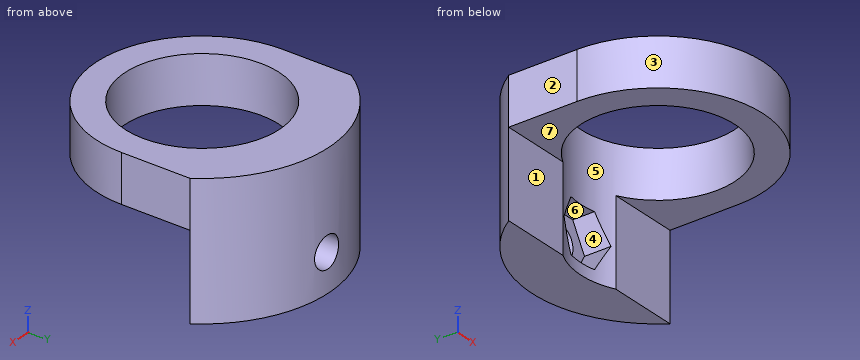
```python
from build123d import *

# Parameters (mm, degrees)
SKETCH1_R               = 8.1
BOSS_EXTRUDE1_DEPTH     = 14
CUT_EXTRUDE1_REACH      = 31.401
SKETCH2_W               = 9
SKETCH2_H               = 18.335502747
CUT_EXTRUDE2_REACH      = 27.601
CUT_EXTRUDE2_END_RADIUS = 13.25
SKETCH3_R               = 1.65
CUT_EXTRUDE3_DEPTH      = 3


with BuildPart() as part:
    # Sketch1 → Boss-Extrude1 (new body)
    with BuildSketch(Plane.XY):
        with BuildLine():
            ThreePointArc((-11.1, 0), (0, -11.1), (11.1, 0))
            Line((11.1, 0), (11.1, 7.235502747))
            ThreePointArc((11.1, 7.235502747), (0, 13.25), (-11.1, 7.235502747))
            Line((-11.1, 7.235502747), (-11.1, 0))
        make_face()
        Circle(SKETCH1_R, mode=Mode.SUBTRACT)
    extrude(amount=BOSS_EXTRUDE1_DEPTH)

    # Cut-Extrude1: up to this face of the body (flat: up to its plane)
    cut_extrude1_end = Plane(part.part.faces().sort_by_distance((11.1, 3.617751373, 7))[0])
    # Sketch2 → Cut-Extrude1 (cut, up to the picked face)
    with BuildSketch(Plane.ZY.offset(11.1), mode=Mode.PRIVATE) as cut_extrude1_sk1:
        with Locations((4.5, -1.932248627)):
            Rectangle(SKETCH2_W, SKETCH2_H)
    cut_extrude1_tool1 = split(extrude(cut_extrude1_sk1.sketch, amount=-CUT_EXTRUDE1_REACH, mode=Mode.PRIVATE), bisect_by=cut_extrude1_end, keep=Keep.BOTH, mode=Mode.PRIVATE)
    add(cut_extrude1_tool1.solids().sort_by(Axis((-11.1, -1.932249, 4.5), (1, 0, 0)))[0], mode=Mode.SUBTRACT)

    # Cut-Extrude2: up to this cylinder (the profile starts inside it)
    cut_extrude2_end = Plane(origin=(0, 0, 4), z_dir=(0, 0, -1)) * Cylinder(CUT_EXTRUDE2_END_RADIUS, 82.702, mode=Mode.PRIVATE)
    # Sketch3 → Cut-Extrude2 (cut, up to the surface)
    with BuildSketch(Plane.XZ.offset(-7.235502747), mode=Mode.PRIVATE) as cut_extrude2_sk1:
        with Locations((0, 4)):
            Circle(SKETCH3_R)
    cut_extrude2_tool1 = extrude(cut_extrude2_sk1.sketch, amount=-CUT_EXTRUDE2_REACH, mode=Mode.PRIVATE) & cut_extrude2_end
    add(cut_extrude2_tool1.solids().sort_by_distance((0, 7.235503, 4))[0], mode=Mode.SUBTRACT)

    # Sketch4 → Cut-Extrude3 (cut)
    with BuildSketch(Plane.XZ.offset(-7.235502747)):
        Polygon((1.616580754, 6.8), (-1.616580754, 6.8), (-3.233161507, 4), (-1.616580754, 1.2), (1.616580754, 1.2), (3.233161507, 4), align=None)
    extrude(amount=-CUT_EXTRUDE3_DEPTH, mode=Mode.SUBTRACT)


solid = part.part
```
Here's how the part is built. I have some questions about the finished solid (model axes, mm). Face numbers are marked on the shaded views. A direction names the side the tool comes from. Round coordinates to 2 decimals unless told otherwise and drop trailing zeros. Loops run counter-clockwise (first coordinate to the right, second up) from the corner with the lowest first, then second, coordinate; pieces in that order, holes last. Notation, with made-up numbers: (44.25, -27) -> (95.25, -27) arc R20 ccw to (95.25, -2) -> close; hole circle Ø2 at (17, 19). An arc over 180 degrees is marked (long way). Answer as CSV lines item,"result". Start each with the question number.
1. Imagine slicing it at B-B on y = 11.25. Write out the boundary of the cut face in (x, z).
2. Imagine slicing it at A-A on x = 0. Write out the boundary of the cut face in (y, z), plus the area to 3 significant figures.
3. If we mould it in two halves opening along X, with no side actions, what happens to the marked faces 1, 2, 3 and 4? For each: pulls with the +X half, pulls with the -X half, needs draft (parallel to the pull), parting line crosses it, or undercut.
4. For the marked faces 5, 6 and 7, which set-ups out of +Z, -Z, +X, -X, +Y, -Y let a thin tool reach every point of the face, with its end or its side?
5. Imagine slicing it at D-D on x = 2.5. Write out the boundary of the cut face in (y, z), plus the area to 3 significant figures.
6. I'm going to push flat-ended pins straight in: P1, Ø4.5, axis at x = 0, z = 4, coming from the -Y side; P2, Ø1.5, axis at x = 8, z = 2.5, coming from the +Y side; P3, Ø3, axis at x = 4, z = 4.5, coming from the -Y side. Where does each tip first touch, or does it pass through?
7. I need wall thicknesses on probe 1 along Y at (x, z) = (0, 9.5); probe 2 along Z at (x, y) = (0, 12.25); probe 3 along Z at (x, y) = (-3, -10). Which ranges of each line are inside material? Lowest first, please. Write a range as from..to.
8. Imagine slicing it at C-C on z = 5. Write out the boundary of the cut face in (x, y).
Solution:
1,outline,"(-7, 0) -> (7, 0) -> (7, 14) -> (-7, 14) -> close; hole circle Ø3.3 at (0, 4)"
2,outline,"(-11.1, 9) -> (-8.1, 9) -> (-8.1, 14) -> (-11.1, 14) -> close; (8.1, 0) -> (13.25, 0) -> (13.25, 2.35) -> (10.24, 2.35) -> (10.24, 1.2) -> (8.1, 1.2) -> close; (8.1, 6.8) -> (10.24, 6.8) -> (10.24, 5.65) -> (13.25, 5.65) -> (13.25, 14) -> (8.1, 14) -> close"
2,area,"65.2 mm²"
3,face 1,"needs draft"
3,face 2,"pulls with the -X half"
3,face 3,"parting line crosses it"
3,face 4,"undercut"
4,face 5,"+Z, -Z"
4,face 6,"-Y"
4,face 7,"-Z, +X, -X, -Y"
5,outline,"(-10.81, 9) -> (-7.7, 9) -> (-7.7, 14) -> (-10.81, 14) -> close; (7.7, 0) -> (13.01, 0) -> (13.01, 14) -> (7.7, 14) -> (7.7, 5.27) -> (10.24, 5.27) -> (10.24, 2.73) -> (7.7, 2.73) -> close"
5,area,"83.4 mm²"
6,P1,"y = 10.24"
6,P2,"y = 11.09"
6,P3,"y = 7.24"
7,probe 1,"-11.1..-8.1, 8.1..13.25"
7,probe 2,"0..2.35, 5.65..14"
7,probe 3,"9..14"
8,outline,"(-11.1, 7.24) -> (-3.64, 7.24) arc R8.1 cw to (-2.66, 7.65) -> (-2.66, 10.24) -> (-1.31, 10.24) -> (-1.31, 13.18) arc R13.25 ccw to start; (1.31, 10.24) -> (2.66, 10.24) -> (2.66, 7.65) arc R8.1 cw to (3.64, 7.24) -> (11.1, 7.24) arc R13.25 ccw to (1.31, 13.18) -> close"
